```python
from build123d import *

# Parameters (mm, degrees)
SKETCH2_W           = 31.75
SKETCH2_H           = 10.16
BOSS_EXTRUDE1_DEPTH = 0.762
SKETCH3_R           = 1.524
SKETCH3_R_2         = 1.8669
CUT_EXTRUDE1_DEPTH  = 1.762
SKETCH4_R           = 0.762
CUT_EXTRUDE2_DEPTH  = 1.762


with BuildPart() as part:
    # Sketch2 → Boss-Extrude1 (new body)
    with BuildSketch(Plane(origin=(0, 0, 0), x_dir=(1, 0, 0), z_dir=(0, 1, 0))):
        Rectangle(SKETCH2_W, SKETCH2_H)
    extrude(amount=BOSS_EXTRUDE1_DEPTH)

    # Sketch3 → Cut-Extrude1 (cut, through all)
    with BuildSketch(Plane(origin=(0, 0.762, 0), x_dir=(1, 0, 0), z_dir=(0, 1, 0))):
        with Locations((-4.191, 0)):
            Circle(SKETCH3_R)
        with Locations((3.7465, 0)):
            Circle(SKETCH3_R_2)
        with Locations((11.684, 0)):
            Circle(SKETCH3_R)
    extrude(amount=-CUT_EXTRUDE1_DEPTH, mode=Mode.SUBTRACT)

    # Sketch4 → Cut-Extrude2 (cut, through all)
    with BuildSketch(Plane(origin=(0, 0.762, 0), x_dir=(1, 0, 0), z_dir=(0, 1, 0))):
        with Locations((-11.938, -2.54)):
            Circle(SKETCH4_R)
    cut_extrude2 = extrude(amount=-CUT_EXTRUDE2_DEPTH, mode=Mode.SUBTRACT)

    # Mirror1: Cut-Extrude2 across plane
    add(cut_extrude2.mirror(Plane.XY), mode=Mode.SUBTRACT)

    # Mirror4: part across plane


with BuildPart() as part_1:
    add(part.part)
    add(part.part.mirror(Plane.ZX))


solid = part_1.part
```
The listing builds one solid part. Answer for the finished solid, in the listing's coordinates (mm). Give positions to 0.01 mm unless a question says otherwise; leave off trailing zeros. Order: outer loops, then holes, each group sorted by start corner. A loop starts at its lowest first (then second) coordinate and runs counter-clockwise, first axis right, second up. Notation, with made-up numbers: (87, -38) -> (120, -38) arc R26 cw to (120, -22) -> close; hole circle Ø1 at (18, 87.5). An arc over 180 degrees is marked (long way). Write each question's results on one line, items separated by ' | '.
Q1. The part is cut by section D-D, the plane z = 2.54. Give the vertices of the cut face in (x, y) (3 decimals).
Checked values:
outline: (-15.875, -0.762) -> (-12.7, -0.762) -> (-12.7, 0.762) -> (-15.875, 0.762) -> close; (-11.176, -0.762) -> (15.875, -0.762) -> (15.875, 0.762) -> (-11.176, 0.762) -> close
Q2. The part is cut by section B-B, the plane x = 10.5. Give the vertices of the cut face in (y, z).
Checked values:
outline: (-0.76, -5.08) -> (0.76, -5.08) -> (0.76, -0.96) -> (-0.76, -0.96) -> close; (-0.76, 0.96) -> (0.76, 0.96) -> (0.76, 5.08) -> (-0.76, 5.08) -> close
Q3. This flat-tipped pin is pushed along its axis until it touches: P1, Ø2.5, axis at x = 11.684, z = 0, coming from the +Y side. Where does it stop, or does it pass through?
Checked values:
P1: passes through
Q4. Straight lines are drawn through the part: probe 1 along X at (y, z) = (0.5, 0) (3 decimals); probe 2 along X at (y, z) = (-0.7, 0.5) (3 decimals); probe 3 along X at (y, z) = (-0.3, -2.54) (3 decimals). For each, find the intervals that lie inside material, in ascending order. Write a range as from..to.
Checked values:
probe 1: x = -15.875..-5.715, -2.667..1.88, 5.613..10.16, 13.208..15.875 | probe 2: x = -15.875..-5.631, -2.751..1.948, 5.545..10.244, 13.124..15.875 | probe 3: x = -15.875..-12.7, -11.176..15.875
Q5. The part is cut by section C-C, the plane z = 0. Give the vertices of the cut face in (x, y) (3 decimals).
Checked values:
outline: (-15.875, -0.762) -> (-5.715, -0.762) -> (-5.715, 0.762) -> (-15.875, 0.762) -> close; (-2.667, -0.762) -> (1.88, -0.762) -> (1.88, 0.762) -> (-2.667, 0.762) -> close; (5.613, -0.762) -> (10.16, -0.762) -> (10.16, 0.762) -> (5.613, 0.762) -> close; (13.208, -0.762) -> (15.875, -0.762) -> (15.875, 0.762) -> (13.208, 0.762) -> close
Q6. The part is cut by section A-A, the plane y = -0.4. Give the vertices of the cut face in (x, z) (1 decimal).
Checked values:
outline: (-15.9, -5.1) -> (15.9, -5.1) -> (15.9, 5.1) -> (-15.9, 5.1) -> close; hole circle Ø1.5 at (-11.9, -2.5); hole circle Ø1.5 at (-11.9, 2.5); hole circle Ø3 at (-4.2, 0); hole circle Ø3.7 at (3.7, 0); hole circle Ø3 at (11.7, 0)
Q7. Determine the mould class of faces 1 (the face through (0, 0, 5.08)), 2 (the face through (-15.875, 0, 0)), 3 (the face through (-2.74, -0.01, -0.46)) for opening direction X: pulls with the +X half, pulls with the -X half, needs draft (parallel to the pull), parting line crosses it, or undercut.
Checked values:
face 1: needs draft | face 2: pulls with the -X half | face 3: undercut
